Could you check a few things on this model? Use its own coordinates, in mm. A direction names the side the tool comes from. Coordinates: 2 decimals unless noted, no trailing zeros. Order: outer loops, then holes, each group sorted by start corner. A loop starts at its lowest first (then second) coordinate and runs counter-clockwise, first axis right, second up. Notation, with made-up numbers: (-5, 7.25) -> (32, 7.25) arc R22 ccw to (32, 19.25) -> close; hole circle Ø11 at (82, 83). An arc over 180 degrees is marked (long way). Use a Markdown table: item, result. Add a question column.
1) If we section it at B-B (z = -12): Write out the boundary of the cut face in (x, y).
2) If we section it at D-D (x = 55.5): Write out the boundary of the cut face in (y, z).
3) If we section it at A-A (x = 121): Write out the boundary of the cut face in (y, z), plus the area to 3 significant figures.
4) Will this pin go through, and if not, where does the flat tip stop? pin 1 Ø12 at (x, z) = (111.5, 6.5) entering from -Y.
5) If we section it at C-C (y = 18): Write out the boundary of the cut face in (x, z).
6) Which directions (+Z, -Z, +X, -X, +Y, -Y) give clear straight access to the entire face, cutting with the end or side of a thin tool? Please do faces 5 (the flat face through (140.233, 199.981, -5.474)), 6 (the flat face through (50.8, 88, 0)), 7 (the flat face through (177.8, 197, -5)).
7) If I drill on L1, parallel to Y at x = 130, z = -0.5; L2, parallel to Y at x = 169, z = 14; L3, parallel to X at y = 118, z = 23, over which ranges is the centre line in solid material (lowest first)? Write a range as [from, to].
8) Thinking about a two-plate mould opening in Z: for faces 1 (the flat face through (140, 209.55, 0)), 2 (the flat face through (101.6, 203, 0)), 3 (the flat face through (48, 141, 25.4)), 4 (the flat face through (113, 177.8, 0)), which applies, +Z half, -Z half, draft (parallel to the pull), parting line (faces both ways), or undercut?
```python
from build123d import *

# Parameters (mm, degrees)
BOSS_EXTRUDE1_DEPTH = 25.4
CUT_EXTRUDE1_DEPTH  = 76.2


with BuildPart() as part:
    # Sketch2 → Boss-Extrude1 (new, symmetric)
    with BuildSketch(Plane.XY):
        Polygon((0, 0), (50.8, 0), (50.8, 177.8), (177.8, 177.8), (177.8, 228.6), (50.8, 228.6), (0, 228.6), align=None)
    extrude(amount=BOSS_EXTRUDE1_DEPTH, both=True)

    # Sketch3 → Cut-Extrude1 (cut)
    with BuildSketch(Plane(origin=(177.8, 0, 0), x_dir=(0, 0, -1), z_dir=(1, 0, 0))):
        Polygon((7.332348419, 203.2), (3.666174209, 209.55), (-3.666174209, 209.55), (-7.332348419, 203.2), (-3.666174209, 196.85), (3.666174209, 196.85), align=None)
    extrude(amount=-CUT_EXTRUDE1_DEPTH, mode=Mode.SUBTRACT)


solid = part.part
```
Answer sheet:
| question | item | result |
|---|---|---|
| 1 | outline | (0, 0) -> (50.8, 0) -> (50.8, 177.8) -> (177.8, 177.8) -> (177.8, 228.6) -> (0, 228.6) -> close |
| 2 | outline | (177.8, -25.4) -> (228.6, -25.4) -> (228.6, 25.4) -> (177.8, 25.4) -> close |
| 3 | outline | (177.8, -25.4) -> (228.6, -25.4) -> (228.6, 25.4) -> (177.8, 25.4) -> close; hole (196.85, -3.67) -> (203.2, -7.33) -> (209.55, -3.67) -> (209.55, 3.67) -> (203.2, 7.33) -> (196.85, 3.67) -> close |
| 3 | area | 2,440 mm2 |
| 4 | pin 1 | y = 177.8 |
| 5 | outline | (0, -25.4) -> (50.8, -25.4) -> (50.8, 25.4) -> (0, 25.4) -> close |
| 6 | face 5 | +X |
| 6 | face 6 | +Z, -Z, +X, -Y |
| 6 | face 7 | +Z, -Z, +X, +Y, -Y |
| 7 | L1 | [177.8, 196.85], [209.55, 228.6] |
| 7 | L2 | [177.8, 228.6] |
| 7 | L3 | [0, 50.8] |
| 8 | face 1 | undercut |
| 8 | face 2 | undercut |
| 8 | face 3 | +Z half |
| 8 | face 4 | draft |
